from build123d import *

# Parameters (mm, degrees)
F0_R     = 2.5
F0_W     = 11.7464
F0_H     = 26.505243
F0_W_2   = 14.56834
F0_H_2   = 30.733124
F1_DEPTH = 4
F2_SIZE  = 2
F4_DEPTH = 56
F5_R     = 3


with BuildPart() as f1:
    # F0 (on Top) → F1 (new body)
    with BuildSketch(Plane.XY):
        with BuildLine():
            ThreePointArc((20, 85), (15.606602, 95.606602), (5, 100))
            Line((5, 100), (-20, 100))
            Line((-20, 100), (-20, -100))
            Line((-20, -100), (5, -100))
            ThreePointArc((5, -100), (15.606602, -95.606602), (20, -85))
            Line((20, -85), (20, 85))
        make_face()
        with Locations((0.5, -83.5)):
            Circle(F0_R, mode=Mode.SUBTRACT)
        with Locations((0.098345, -35.93968)):
            Rectangle(F0_W, F0_H, mode=Mode.SUBTRACT)
        with Locations((0.947373, 0)):
            Rectangle(F0_W_2, F0_H_2, mode=Mode.SUBTRACT)
        with Locations((0.098345, 35.93968)):
            Rectangle(F0_W, F0_H, mode=Mode.SUBTRACT)
        with Locations((0.5, 83.5)):
            Circle(F0_R, mode=Mode.SUBTRACT)
    extrude(amount=-F1_DEPTH)

    # F2
    f2_edges = [f1.edges().sort_by_distance(p)[0] for p in [
        (-2, -83.5, 0),
        (-2, 83.5, 0),
    ]]
    chamfer(f2_edges, length=F2_SIZE)

    # F3 (on Front) → F4 (join, symmetric)
    with BuildSketch(Plane.XZ):
        with BuildLine():
            Line((8.001845, -20.259996), (8.01102, -6.651434))
            Line((8.01102, -6.651434), (10.020183, -3.892345))
            Line((10.020183, -3.892345), (7.950272, -3.389892))
            Line((7.950272, -3.389892), (6.068421, -6.165784))
            Line((6.068421, -6.165784), (6.245231, -19.775091))
            ThreePointArc((6.245231, -19.775091), (5.774018, -20.746688), (4.723544, -20.996785))
            Line((4.723544, -20.996785), (-7.11199, -20.996785))
            ThreePointArc((-7.11199, -20.996785), (-7.875169, -20.761546), (-8.37348, -20.137473))
            Line((-8.37348, -20.137473), (-8.37348, -4))
            Line((-8.37348, -4), (-10.235702, -4))
            Line((-10.235702, -4), (-10.235702, -20.073208))
            ThreePointArc((-10.235702, -20.073208), (-9.544714, -22.146454), (-7.563292, -23.068289))
            Line((-7.563292, -23.068289), (6.496039, -22.776224))
            ThreePointArc((6.496039, -22.776224), (7.596641, -21.726186), (8.001845, -20.259996))
        make_face()
    extrude(amount=F4_DEPTH, both=True)

    # F5
    f5_edges = [f1.edges().sort_by_distance(p)[0] for p in [
        (-20, 0, 0),
    ]]
    fillet(f5_edges, radius=F5_R)


solid = f1.part
CAD build for the part. Positions are in the model's coordinates, mm. A direction names the side the tool comes from. Coordinates: 2 decimals unless noted, no trailing zeros. Write each loop counter-clockwise with the first axis right and the second up, starting at its lowest first coordinate (ties: lowest second). Pieces come first, ordered by that corner, then holes. Notation, with made-up numbers: (89.5, 34) - (118.5, 34) arc R18 ccw to (118.5, 40) - close; hole circle Ø9 at (-23, 81.5). An arc over 180 degrees is marked (long way). Use a Markdown table: item, result. Add a question column.
Item 1: Band-saw the part on A-A, the plane x = 0.5. Give the number of separate pieces and of enclosed holes in the cut face, and give its area (3 significant figures).
Item 2: Band-saw the part on B-B, the plane z = -17.75. Give the cut face in (x, y), and give its area (3 significant figures).
Item 3: Band-saw the part on C-C, the plane y = -68. Give the cut face in (x, z), and give its area (3 significant figures).
Item 4: 3-axis set-ups, long thin cutter, end or side, ignore diameter. For faces 1 (the face through (20, -1, -2)), 2 (the face through (-0.9, 56, -21.3)), 3 (the face through (-6.337, 0, -2)), 4 (the face through (-10.236, -1, -12)), 5 (the face through (0.17, 85.98, -2.99)): which of +Z, -Z, +X, -X, +Y, -Y reach the whole face in a straight line?
Item 5: Drill centre lines: L1, parallel to Y at x = 0.5, z = -3.2; L2, parallel to X at y = -4.5, z = -20; L3, parallel to Z at x = -11, y = 80.5. Where is each one in solid material? Low to high. Write a range as from..to.
Item 6: Band-saw the part on D-D, the plane y = 19. Give the cut face in (x, z).
Item 7: Flat gauge pins, fed straight in: pin 1 (5 mm diameter, centred on y = 12.5, z = -15.5, fed in from -X); pin 2 (5 mm diameter, centred on x = -13, y = -70.5, fed in from -Z); pin 3 (6 mm diameter, centred on x = 9.5, z = -13.5, fed in from +Y). Where does each tip first touch, or does it go through?
Item 8: Mould opens along Z. For faces 6 (the face through (-8.373, -1, -12)), 7 (the face through (15.72, 95.49, -1.97)), 8 (the face through (9, 1, 0)) say: pulls with the +Z half, pulls with the -Z half, needs draft (parallel to the pull), parting line crosses it, or undercut.
Numbers:
| question | item | result |
|---|---|---|
| 1 | separate pieces | 7 |
| 1 | enclosed holes | 0 |
| 1 | area | 630 mm2 |
| 2 | outline | (-10.24, -56) - (-8.37, -56) - (-8.37, 56) - (-10.24, 56) - close; (6.22, -56) - (8, -56) - (8, 56) - (6.22, 56) - close |
| 2 | area | 408 mm2 |
| 3 | outline | (-20, -4) - (20, -4) - (20, 0) - (-17, 0) arc R3 ccw to (-20, -3) - close |
| 3 | area | 158 mm2 |
| 4 | face 1 | +Z, -Z, +X, +Y, -Y |
| 4 | face 2 | -Z, +X, -X, +Y |
| 4 | face 3 | +Z |
| 4 | face 4 | -Z, -X, +Y, -Y |
| 4 | face 5 | +Z, -Z |
| 5 | L1 | -100..-86, -81..-49.19, -22.69..-15.37, 15.37..22.69, 49.19..81, 86..100 |
| 5 | L2 | -10.24..-8.37, 6.22..8 |
| 5 | L3 | -4..0 |
| 6 | outline | (-20, -4) - (-10.24, -4) - (-10.24, -20.07) arc R2.76 ccw to (-7.56, -23.07) - (6.5, -22.78) arc R2.86 ccw to (8, -20.26) - (8.01, -6.65) - (9.94, -4) - (20, -4) - (20, 0) - (-17, 0) arc R3 ccw to (-20, -3) - close; hole (-8.37, -20.14) arc R1.36 ccw to (-7.11, -21) - (4.72, -21) arc R1.26 ccw to (6.25, -19.78) - (6.07, -6.17) - (7.54, -4) - (-8.37, -4) - close |
| 7 | pin 1 | x = -10.24 |
| 7 | pin 2 | z = -4 |
| 7 | pin 3 | y = 56 |
| 8 | face 6 | undercut |
| 8 | face 7 | needs draft |
| 8 | face 8 | pulls with the +Z half |
